Could you check a few things on this model? Use its own coordinates, in mm. Round coordinates to 2 decimals unless told otherwise and drop trailing zeros. Write each loop counter-clockwise with the first axis right and the second up, starting at its lowest first coordinate (ties: lowest second). Pieces come first, ordered by that corner, then holes.
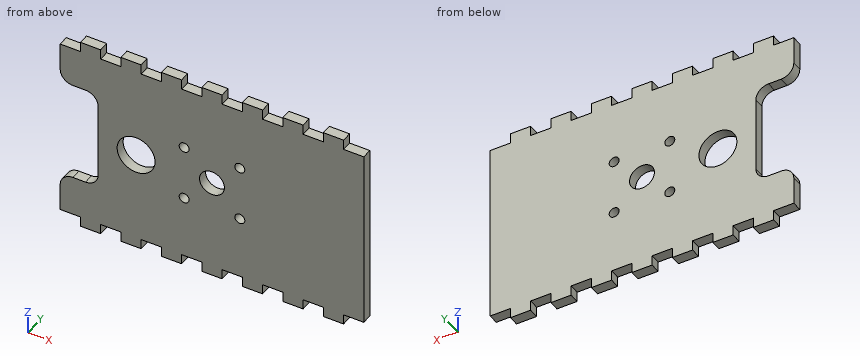
Autodesk Inventor part; units mm, degrees
ref_plane "YZ Plane" through (0, 0, 0) normal (1, 0, 0) x (0, 1, 0)
ref_plane "XZ Plane" through (0, 0, 0) normal (0, 1, 0) x (-1, 0, 0)
ref_plane "XY Plane" through (0, 0, 0) normal (0, 0, 1) x (1, 0, 0)
sketch "Sketch1" plane through (0, 0, 0) normal (0, 1, 0) x (-1, 0, 0)
  line L0 (-76.2, 50.8) -> (76.2, 50.8)
  line L1 (76.2, 50.8) -> (76.2, -50.8)
  line L2 (76.2, -50.8) -> (-76.2, -50.8)
  line L3 (-76.2, -50.8) -> (-76.2, 50.8)
  line L4 (-76.2, 50.8) -> (76.2, -50.8) construction
  line L5 (76.2, 50.8) -> (-76.2, -50.8) construction
  point P0 (0, 0)
  dimension "d0" = 152.4
  dimension "d1" = 101.6
extrude "Extrusion1" add sketch "Sketch1" along normal blind 5.08
sketch "Sketch2" plane through (0, 5.08, 0) normal (0, 1, 0) x (1, 0, 0)
  line L0 (-76.2, -50.8) -> (76.2, -50.8)
  line L1 (76.2, -50.8) -> (76.2, 50.8)
  line L2 (76.2, 50.8) -> (-76.2, 50.8)
  line L3 (-76.2, 50.8) -> (-76.2, -50.8)
  line L4 (-76.2, -50.8) -> (-66.04, -50.8)
  line L5 (-66.04, -50.8) -> (-66.04, -45.72)
  line L6 (-66.04, -45.72) -> (-76.2, -45.72)
  line L7 (-76.2, -45.72) -> (-76.2, -50.8)
  line L8 (-55.88, -50.8) -> (-45.72, -50.8)
  line L9 (-45.72, -50.8) -> (-45.72, -45.72)
  line L10 (-45.72, -45.72) -> (-55.88, -45.72)
  line L11 (-55.88, -45.72) -> (-55.88, -50.8)
  line L12 (-35.56, -50.8) -> (-25.4, -50.8)
  line L13 (-25.4, -50.8) -> (-25.4, -45.72)
  line L14 (-25.4, -45.72) -> (-35.56, -45.72)
  line L15 (-35.56, -45.72) -> (-35.56, -50.8)
  line L16 (-15.24, -50.8) -> (-5.08, -50.8)
  line L17 (-5.08, -50.8) -> (-5.08, -45.72)
  line L18 (-5.08, -45.72) -> (-15.24, -45.72)
  line L19 (-15.24, -45.72) -> (-15.24, -50.8)
  line L20 (5.08, -50.8) -> (15.24, -50.8)
  line L21 (15.24, -50.8) -> (15.24, -45.72)
  line L22 (15.24, -45.72) -> (5.08, -45.72)
  line L23 (5.08, -45.72) -> (5.08, -50.8)
  line L24 (25.4, -50.8) -> (35.56, -50.8)
  line L25 (35.56, -50.8) -> (35.56, -45.72)
  line L26 (35.56, -45.72) -> (25.4, -45.72)
  line L27 (25.4, -45.72) -> (25.4, -50.8)
  line L28 (45.72, -50.8) -> (55.88, -50.8)
  line L29 (55.88, -50.8) -> (55.88, -45.72)
  line L30 (55.88, -45.72) -> (45.72, -45.72)
  line L31 (45.72, -45.72) -> (45.72, -50.8)
  line L32 (66.04, -50.8) -> (76.2, -50.8)
  line L33 (76.2, -50.8) -> (76.2, -45.72)
  line L34 (76.2, -45.72) -> (66.04, -45.72)
  line L35 (66.04, -45.72) -> (66.04, -50.8)
  line L36 (-76.2, 50.8) -> (-76.2, -50.8) construction
  line L37 (-76.2, 0) -> (76.2, 0) construction
  line L38 (-76.2, 50.8) -> (76.2, 50.8)
  line L39 (-76.2, 50.8) -> (-66.04, 50.8)
  line L40 (-66.04, 50.8) -> (-66.04, 45.72)
  line L41 (-66.04, 45.72) -> (-76.2, 45.72)
  line L42 (-76.2, 45.72) -> (-76.2, 50.8)
  line L43 (-55.88, 50.8) -> (-45.72, 50.8)
  line L44 (-45.72, 50.8) -> (-45.72, 45.72)
  line L45 (-45.72, 45.72) -> (-55.88, 45.72)
  line L46 (-55.88, 45.72) -> (-55.88, 50.8)
  line L47 (-35.56, 50.8) -> (-25.4, 50.8)
  line L48 (-25.4, 50.8) -> (-25.4, 45.72)
  line L49 (-25.4, 45.72) -> (-35.56, 45.72)
  line L50 (-35.56, 45.72) -> (-35.56, 50.8)
  line L51 (-15.24, 50.8) -> (-5.08, 50.8)
  line L52 (-5.08, 50.8) -> (-5.08, 45.72)
  line L53 (-5.08, 45.72) -> (-15.24, 45.72)
  line L54 (-15.24, 45.72) -> (-15.24, 50.8)
  line L55 (5.08, 50.8) -> (15.24, 50.8)
  line L56 (15.24, 50.8) -> (15.24, 45.72)
  line L57 (15.24, 45.72) -> (5.08, 45.72)
  line L58 (5.08, 45.72) -> (5.08, 50.8)
  line L59 (25.4, 50.8) -> (35.56, 50.8)
  line L60 (35.56, 50.8) -> (35.56, 45.72)
  line L61 (35.56, 45.72) -> (25.4, 45.72)
  line L62 (25.4, 45.72) -> (25.4, 50.8)
  line L63 (45.72, 50.8) -> (55.88, 50.8)
  line L64 (55.88, 50.8) -> (55.88, 45.72)
  line L65 (55.88, 45.72) -> (45.72, 45.72)
  line L66 (45.72, 45.72) -> (45.72, 50.8)
  line L67 (66.04, 50.8) -> (76.2, 50.8)
  line L68 (76.2, 50.8) -> (76.2, 45.72)
  line L69 (76.2, 45.72) -> (66.04, 45.72)
  line L70 (66.04, 45.72) -> (66.04, 50.8)
  point P0 (0, 0)
  point P1 (0, 0)
  dimension "d11" = 10.16
  dimension "d12" = 5.08
  dimension "d13" = 0
  dimension "d16" = 20.32
hole "Hole1" at (0, 5.08, 0) direction (0, -1, 0) diameter 12.5 end through all
extrude "Extrusion2" cut sketch "Sketch2" against normal blind 5.08 contours L5 L6 L3 L41 L40 L2 L46 L45 L44 L50 L49 L48 L54 L53 L52 L58 L57 L56 L62 L61 L60 L66 L65 L64 L70 L69 L1 L34 L35 L0 L29 L30 L31 L25 L26 L27 L21 L22 L23 L17 L18 L19 L13 L14 L15 L9 L10 L11 keep common part
sketch "Sketch3" plane through (0, 0, 0) normal (0, -1, 0) x (1, 0, 0)
  circle A0 centre (-38.1, 0) radius 9.525
  line L0 (0, 0) -> (-38.1, 0) construction
  dimension "d23" = 19.05
  dimension "d24" = 38.1
extrude "Extrusion3" cut sketch "Sketch3" against normal blind 25.4
sketch "Sketch4" plane through (0, 0, 0) normal (0, -1, 0) x (1, 0, 0)
  circle A0 centre (13.97, -13.97) radius 2.5
  circle A1 centre (-13.97, -13.97) radius 2.5
  circle A2 centre (-13.97, 13.97) radius 2.5
  circle A3 centre (13.97, 13.97) radius 2.5
  point P0 (0, 0)
extrude "Extrusion4" cut sketch "Sketch4" against normal blind 25.4
sketch "Sketch5" plane through (0, 0, 0) normal (0, -1, 0) x (1, 0, 0)
  circle A0 centre (-13.97, 13.97) radius 2.5
  circle A1 centre (13.97, -13.97) radius 2.5
  circle A2 centre (-13.97, -13.97) radius 2.5
  circle A3 centre (13.97, 13.97) radius 2.5
  circle A4 centre (-38.1, 0) radius 9.525
  circle A5 centre (0, 0) radius 6.25
  line L0 (66.04, -45.72) -> (66.04, -50.8) construction
  line L1 (76.2, -45.72) -> (66.04, -45.72) construction
  line L2 (76.2, -45.72) -> (76.2, 45.72) construction
  line L3 (66.04, 45.72) -> (76.2, 45.72) construction
  line L4 (66.04, 50.8) -> (66.04, 45.72) construction
  line L5 (66.04, 50.8) -> (55.88, 50.8) construction
  line L6 (55.88, 45.72) -> (55.88, 50.8) construction
  line L7 (45.72, 45.72) -> (55.88, 45.72) construction
  line L8 (45.72, 50.8) -> (45.72, 45.72) construction
  line L9 (45.72, 50.8) -> (35.56, 50.8) construction
  line L10 (35.56, 45.72) -> (35.56, 50.8)
  line L11 (25.4, 45.72) -> (35.56, 45.72)
  line L12 (25.4, 50.8) -> (25.4, 45.72)
  line L13 (25.4, 50.8) -> (15.24, 50.8)
  line L14 (15.24, 45.72) -> (15.24, 50.8)
  line L15 (5.08, 45.72) -> (15.24, 45.72)
  line L16 (5.08, 50.8) -> (5.08, 45.72)
  line L17 (5.08, 50.8) -> (-5.08, 50.8)
  line L18 (-5.08, 45.72) -> (-5.08, 50.8)
  line L19 (-15.24, 45.72) -> (-5.08, 45.72)
  line L20 (-15.24, 50.8) -> (-15.24, 45.72)
  line L21 (-15.24, 50.8) -> (-25.4, 50.8)
  line L22 (-25.4, 45.72) -> (-25.4, 50.8)
  line L23 (-35.56, 45.72) -> (-25.4, 45.72)
  line L24 (-35.56, 50.8) -> (-35.56, 45.72)
  line L25 (-35.56, 50.8) -> (-45.72, 50.8)
  line L26 (-45.72, 45.72) -> (-45.72, 50.8)
  line L27 (-55.88, 45.72) -> (-45.72, 45.72)
  line L28 (-55.88, 50.8) -> (-55.88, 45.72)
  line L29 (-55.88, 50.8) -> (-66.04, 50.8)
  line L30 (-66.04, 45.72) -> (-66.04, 50.8)
  line L31 (-76.2, 45.72) -> (-66.04, 45.72)
  line L32 (-76.2, 45.72) -> (-76.2, -45.72)
  line L33 (-66.04, -45.72) -> (-76.2, -45.72)
  line L34 (-66.04, -50.8) -> (-66.04, -45.72)
  line L35 (-66.04, -50.8) -> (-55.88, -50.8)
  line L36 (-55.88, -45.72) -> (-55.88, -50.8)
  line L37 (-45.72, -45.72) -> (-55.88, -45.72)
  line L38 (-45.72, -50.8) -> (-45.72, -45.72)
  line L39 (-45.72, -50.8) -> (-35.56, -50.8)
  line L40 (-35.56, -45.72) -> (-35.56, -50.8)
  line L41 (-25.4, -45.72) -> (-35.56, -45.72)
  line L42 (-25.4, -50.8) -> (-25.4, -45.72)
  line L43 (-25.4, -50.8) -> (-15.24, -50.8)
  line L44 (-15.24, -45.72) -> (-15.24, -50.8)
  line L45 (-5.08, -45.72) -> (-15.24, -45.72)
  line L46 (-5.08, -50.8) -> (-5.08, -45.72)
  line L47 (-5.08, -50.8) -> (5.08, -50.8)
  line L48 (5.08, -45.72) -> (5.08, -50.8)
  line L49 (15.24, -45.72) -> (5.08, -45.72)
  line L50 (15.24, -50.8) -> (15.24, -45.72)
  line L51 (15.24, -50.8) -> (25.4, -50.8)
  line L52 (25.4, -45.72) -> (25.4, -50.8)
  line L53 (35.56, -45.72) -> (25.4, -45.72)
  line L54 (35.56, -50.8) -> (35.56, -45.72)
  line L55 (35.56, -50.8) -> (45.72, -50.8) construction
  line L56 (45.72, -45.72) -> (45.72, -50.8) construction
  line L57 (55.88, -45.72) -> (45.72, -45.72) construction
  line L58 (55.88, -50.8) -> (55.88, -45.72) construction
  line L59 (55.88, -50.8) -> (66.04, -50.8) construction
  line L60 (-76.2, -45.72) -> (-76.2, 45.72)
  line L61 (-76.2, 25.4) -> (-57.15, 25.4)
  line L62 (-57.15, 25.4) -> (-57.15, -25.4)
  line L63 (-57.15, -25.4) -> (-76.2, -25.4)
  line L64 (-76.2, -25.4) -> (-76.2, 25.4)
  line L65 (-57.15, 0) -> (-76.2, 0) construction
  line L66 (-76.2, 25.4) -> (-57.15, 25.4)
  line L67 (-57.15, 25.4) -> (-57.15, -25.4)
  line L68 (-57.15, -25.4) -> (-76.2, -25.4)
  line L69 (-76.2, -25.4) -> (-76.2, 25.4)
  dimension "d29" = 50.8
  dimension "d30" = 19.05
extrude "Extrusion5" cut sketch "Sketch5" against normal blind 25.4 contours L61 L62 L63 L32
fillet "Fillet1" radius 6.35 4 edges at (-57.15, 2.54, -25.4) (-76.2, 2.54, -25.4) (-57.15, 2.54, 25.4) (-76.2, 2.54, 25.4)
properties part number "ArmMount" material "Wood (Birch)"
Q1. If I drill on L1, parallel to Z at x = -13.97, y = 3.7; L2, parallel to Z at x = -38.1, y = 3.7 (3 decimals); L3, parallel to X at y = 2.7, z = -15.5, over which ranges is the centre line in solid material (lowest first)?
Q2. I'm going to push flat-ended pins straight in: pin 1 Ø1.5 at (y, z) = (2.5, -49) entering from -X; pin 2 Ø1.5 at (x, z) = (-24.5, 35.5) entering from -Y; pin 3 Ø2.5 at (x, y) = (72.5, 3) entering from +Z; pin 4 Ø1 at (y, z) = (0.5, -30.5) entering from -X. Where does each tip first touch, or does it pass through?
Q3. Imagine slicing it at C-C, the plane y = 3.5. Count the separate pieces of the cut face and the enclosed holes in it, then the cut area to 3 significant figures.
Q4. Imagine slicing it at B-B, the plane z = 0. Write out the boundary of the cut face in (x, y) (3 decimals).
Q5. Imagine slicing it at A-A, the plane z = -13.97. Write out the boundary of the cut face in (x, y).
Results found:
1. L1: z = -45.72 to -16.47, -11.47 to 11.47, 16.47 to 45.72
1. L2: z = -50.8 to -9.525, 9.525 to 50.8
1. L3: x = -57.15 to -15.95, -11.99 to 11.99, 15.95 to 76.2
2. pin 1: stops at x = -66.04
2. pin 2: stops at y = 0
2. pin 3: stops at z = 45.72
2. pin 4: stops at x = -76.16
3. separate pieces: 1
3. enclosed holes: 6
3. area: 13,200 mm2
4. outline: (-57.15, 0) - (-47.625, 0) - (-47.625, 5.08) - (-57.15, 5.08) - close; (-28.575, 0) - (-6.25, 0) - (-6.25, 5.08) - (-28.575, 5.08) - close; (6.25, 0) - (76.2, 0) - (76.2, 5.08) - (6.25, 5.08) - close
5. outline: (-57.15, 0) - (-16.47, 0) - (-16.47, 5.08) - (-57.15, 5.08) - close; (-11.47, 0) - (11.47, 0) - (11.47, 5.08) - (-11.47, 5.08) - close; (16.47, 0) - (76.2, 0) - (76.2, 5.08) - (16.47, 5.08) - close
